Work out the finished part from the listing and answer in its coordinate system (mm). Face numbers are marked on the shaded views. A direction names the side the tool comes from. Give positions to 0.01 mm unless a question says otherwise; leave off trailing zeros. Loops run counter-clockwise (first coordinate to the right, second up) from the corner with the lowest first, then second, coordinate; pieces in that order, holes last. Notation, with made-up numbers: (33.25, -1) -> (74.25, -1) arc R29 cw to (74.25, 24) -> close; hole circle Ø3 at (88.25, 22). An arc over 180 degrees is marked (long way). Answer as CSV lines item,"result". Start each with the question number.
1. Find section D-D, the plane z = 35.5. Give the vertices of the cut face in (x, y) (3 decimals).
2. Flat-ended cylindrical pins translate along their axes: pin 1 Ø1 at (x, z) = (9.5, 22.5) entering from -Y; pin 2 Ø4 at (y, z) = (-13, 16.5) entering from -X; pin 3 Ø6 at (x, z) = (-0.5, 16) entering from -Y (3 decimals). Find the tip coordinate at first contact, or state that the pin passes through.
3. Find section A-A, the plane x = 0. Give the vertices of the cut face in (y, z) (1 decimal).
4. Find the intervals of material crossed by line 1 along Y through (x, z) = (0, 17.75) (1 decimal); line 2 along Y through (x, z) = (0, 44.75) (1 decimal), in increasing order.
5. Find section C-C, the plane z = 45. Give the vertices of the cut face in (x, y) (1 decimal), and give its area (3 significant figures).
6. Determine the mould class of the marked faces 1, 2 and 3 for opening direction Y: +Y half, -Y half, draft (parallel to the pull), parting line (faces both ways), or undercut.
7. A tool of negligible diameter and unlimited length cuts with its end or side. For the marked faces 4 and 5, from which of +Z, -Z, +X, -X, +Y, -Y can it reach the whole face along a straight path? Write none if from no direction.
from build123d import *

# Parameters (mm, degrees)
F2_R     = 4.7625
F3_DEPTH = 9.525
F4_R     = 1.5875
F5_DEPTH = 22.225


with BuildPart() as f1:
    # F0 (on Front) → F1 (revolve)
    with BuildSketch(Plane.XZ):
        Polygon((3.81, 1.888357), (31.115, 12.7), (31.115, 25.4), (6.985, 25.4), (6.985, 50.8), (0, 50.8), (0, 1.888357), align=None)
    revolve(axis=Axis((0, 0, 26.344178), (0, 0, -1)))

    # F2 (on face) → F3 (cut)
    with BuildSketch(Plane.XY.offset(50.8)):
        Circle(F2_R)
    extrude(amount=-F3_DEPTH, mode=Mode.SUBTRACT)

    # F4 (on face) → F5 (cut)
    with BuildSketch(Plane(origin=(0, 0, 1.888357), x_dir=(1, 0, 0), z_dir=(0, 0, -1))):
        Circle(F4_R)
    extrude(amount=-F5_DEPTH, mode=Mode.SUBTRACT)


solid = f1.part
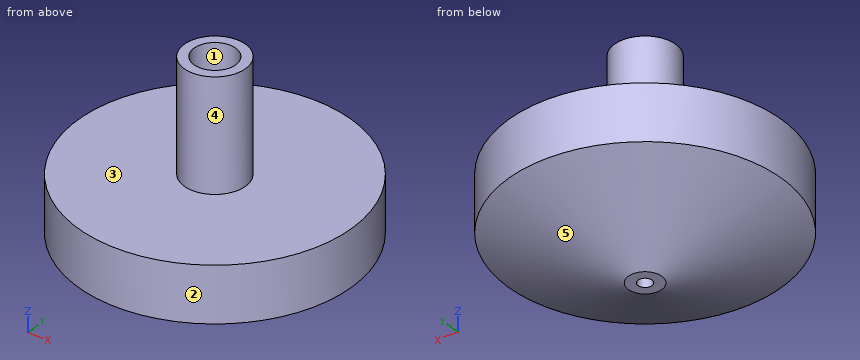
Resolved:
1,outline,"circle Ø13.97 at (0, 0)"
2,pin 1,"stops at y = -29.78"
2,pin 2,"stops at x = -29.11"
2,pin 3,"stops at y = -31.115"
3,outline,"(-31.1, 12.7) -> (-3.8, 1.9) -> (-1.6, 1.9) -> (-1.6, 24.1) -> (1.6, 24.1) -> (1.6, 1.9) -> (3.8, 1.9) -> (31.1, 12.7) -> (31.1, 25.4) -> (7, 25.4) -> (7, 50.8) -> (4.8, 50.8) -> (4.8, 41.3) -> (-4.8, 41.3) -> (-4.8, 50.8) -> (-7, 50.8) -> (-7, 25.4) -> (-31.1, 25.4) -> close"
4,line 1,"y = -31.1 to -1.6, 1.6 to 31.1"
4,line 2,"y = -7 to -4.8, 4.8 to 7"
5,outline,"circle Ø14 at (0, 0); hole circle Ø9.5 at (0, 0)"
5,area,"82.0 mm^2"
6,face 1,"undercut"
6,face 2,"parting line"
6,face 3,"draft"
7,face 4,"+Z"
7,face 5,"-Z"
